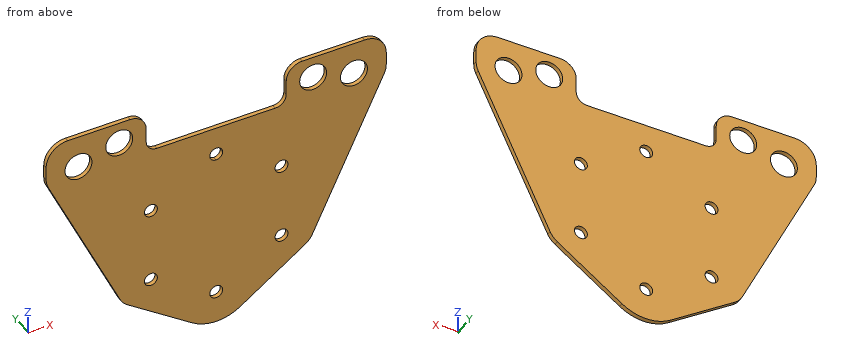
```python
from build123d import *

# Parameters (mm, degrees)
F1_R     = 3
F1_R_2   = 6.25
F2_DEPTH = 2


with BuildPart() as f2:
    # F1 (on Front) → F2 (new body)
    with BuildSketch(Plane.XZ):
        with BuildLine():
            Line((-41.189004, -26.319483), (-11.225195, -46.63929))
            ThreePointArc((-11.225195, -46.63929), (0, -50.086496), (11.225195, -46.63929))
            Line((11.225195, -46.63929), (41.189004, -26.319483))
            ThreePointArc((41.189004, -26.319483), (43.148737, -24.574534), (44.587085, -22.379868))
            Line((44.587085, -22.379868), (77.928371, 46.894439))
            ThreePointArc((77.928371, 46.894439), (78.667226, 49.007124), (78.917693, 51.231222))
            Line((78.917693, 51.231222), (78.917693, 57.371839))
            ThreePointArc((78.917693, 57.371839), (75.988761, 64.442907), (68.917693, 67.371839))
            Line((68.917693, 67.371839), (39.985476, 67.371839))
            ThreePointArc((39.985476, 67.371839), (34.682175, 65.17514), (32.485476, 59.871839))
            Line((32.485476, 59.871839), (32.485476, 53.130572))
            ThreePointArc((32.485476, 53.130572), (31.02101, 49.595038), (27.485476, 48.130572))
            Line((27.485476, 48.130572), (0, 48.130572))
            Line((0, 48.130572), (-27.485476, 48.130572))
            ThreePointArc((-27.485476, 48.130572), (-31.02101, 49.595038), (-32.485476, 53.130572))
            Line((-32.485476, 53.130572), (-32.485476, 59.871839))
            ThreePointArc((-32.485476, 59.871839), (-34.682175, 65.17514), (-39.985476, 67.371839))
            Line((-39.985476, 67.371839), (-68.917693, 67.371839))
            ThreePointArc((-68.917693, 67.371839), (-75.988761, 64.442907), (-78.917693, 57.371839))
            Line((-78.917693, 57.371839), (-78.917693, 51.231222))
            ThreePointArc((-78.917693, 51.231222), (-78.667226, 49.007124), (-77.928371, 46.894439))
            Line((-77.928371, 46.894439), (-44.587085, -22.379868))
            ThreePointArc((-44.587085, -22.379868), (-43.148737, -24.574534), (-41.189004, -26.319483))
        make_face()
        with Locations((-30.310889, -17.5)):
            Circle(F1_R, mode=Mode.SUBTRACT)
        with Locations((0, -35)):
            Circle(F1_R, mode=Mode.SUBTRACT)
        with Locations((30.310889, -17.5)):
            Circle(F1_R, mode=Mode.SUBTRACT)
        with Locations((-30.310889, 17.5)):
            Circle(F1_R, mode=Mode.SUBTRACT)
        with Locations((-63.917693, 52.371839)):
            Circle(F1_R_2, mode=Mode.SUBTRACT)
        with Locations((-45, 57.371839)):
            Circle(F1_R_2, mode=Mode.SUBTRACT)
        with Locations((30.310889, 17.5)):
            Circle(F1_R, mode=Mode.SUBTRACT)
        with BuildLine():
            ThreePointArc((0, 32), (-2.12132, 37.12132), (3, 35))
            ThreePointArc((3, 35), (2.12132, 32.87868), (0, 32))
        make_face(mode=Mode.SUBTRACT)
        with Locations((63.917693, 52.371839)):
            Circle(F1_R_2, mode=Mode.SUBTRACT)
        with Locations((45, 57.371839)):
            Circle(F1_R_2, mode=Mode.SUBTRACT)
    extrude(amount=-F2_DEPTH)


solid = f2.part
```
Could you check a few things on this model? Use its own coordinates, in mm. Coordinates: 2 decimals unless noted, no trailing zeros. Loops run counter-clockwise (first coordinate to the right, second up) from the corner with the lowest first, then second, coordinate; pieces in that order, holes last. Notation, with made-up numbers: M 29,46.5 L 52,46.5 A19 ccw 52,58.5 Z; hole C -9.5,-13.75 d1. An arc over 180 degrees is marked long. Put each result on its own line as item: value. Start each with the question number.
(1) Suppose I cut it at A-A on z = 17.5. Please give me the cut outline in (x, y), then the cut area to 3 significant figures.
(2) Suppose I cut it at D-D on z = 44. Please give me the cut outline in (x, y).
(3) I need wall thicknesses on line 1 (X direction, y = 1.75, z = 16); line 2 (X direction, y = 0.7, z = 49); line 3 (Z direction, x = -41.5, y = 0.5). Which ranges of each line are inside material? Lowest first, please. Write a range as from..to.
(4) Will this pin go through, and if not, where does the flat tip stop? P1, Ø16, axis at x = 63.92, z = 52.37, coming from the -Y side.
(5) Suppose I cut it at C-C on y = 0.8. Count the separate pieces of the cut face and the enclosed holes in it, then the cut area to 3 significant figures.
(6) Suppose I cut it at B-B on z = -35. Please give me the cut outline in (x, y), then the cut area to 3 significant figures.
Solutions:
1. outline: M -63.78,0 L -33.31,0 L -33.31,2 L -63.78,2 Z; M -27.31,0 L 27.31,0 L 27.31,2 L -27.31,2 Z; M 33.31,0 L 63.78,0 L 63.78,2 L 33.31,2 Z
1. area: 231 mm2
2. outline: M -76.54,0 L 76.54,0 L 76.54,2 L -76.54,2 Z
3. line 1: x = -63.06..-32.91, -27.71..27.71, 32.91..63.06
3. line 2: x = -78.67..-69.18, -58.66..-30.3, 30.3..58.66, 69.18..78.67
3. line 3: z = -26.1..52.19, 62.55..67.37
4. P1: stops at y = 0
5. separate pieces: 1
5. enclosed holes: 10
5. area: 11,200 mm2
6. outline: M -28.39,0 L -3,0 L -3,2 L -28.39,2 Z; M 3,0 L 28.39,0 L 28.39,2 L 3,2 Z
6. area: 102 mm2
